Geometry: see drawing. Coordinates: mm, zero at the bounding-box minimum. Round coordinates to 2 decimals unless told otherwise and drop trailing zeros. Order: outer loops, then holes, each group sorted by start corner. A loop starts at its lowest first (then second) coordinate and runs counter-clockwise, first axis right, second up. Notation, with made-up numbers: (-15, 46) -> (22, 46) arc R37 ccw to (22, 85) -> close; hole circle Ø5 at (43.25, 38.25). An arc over 180 degrees is marked (long way). Put each result on its own line as item: value.
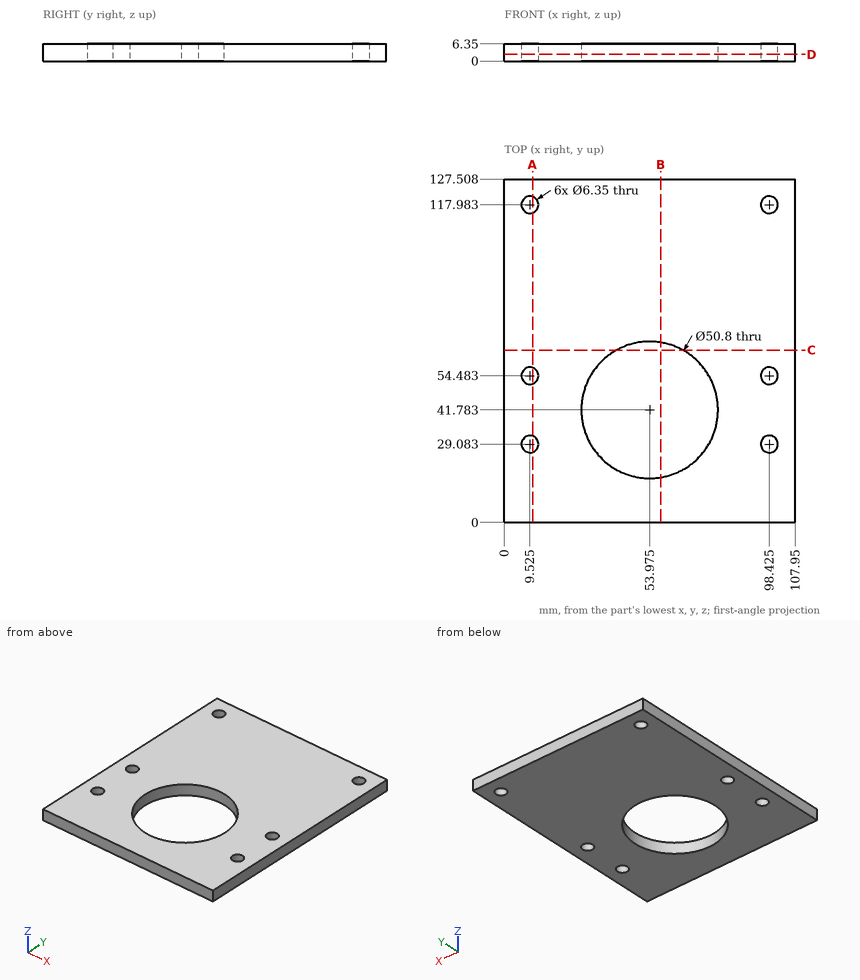
1. Cut plane B-B on x = 58. Return loops of the section in (y, z).
Ans:
outline: (0, 0) -> (16.7, 0) -> (16.7, 6.35) -> (0, 6.35) -> close; (66.86, 0) -> (127.51, 0) -> (127.51, 6.35) -> (66.86, 6.35) -> close
2. Cut plane C-C on y = 64. Return loops of the section in (x, z), and give its area (3 significant figures).
Ans:
outline: (0, 0) -> (41.66, 0) -> (41.66, 6.35) -> (0, 6.35) -> close; (66.29, 0) -> (107.95, 0) -> (107.95, 6.35) -> (66.29, 6.35) -> close
area: 529 mm²
3. Cut plane A-A on x = 10.5. Return loops of the section in (y, z), and give its area (3 significant figures).
Ans:
outline: (0, 0) -> (26.06, 0) -> (26.06, 6.35) -> (0, 6.35) -> close; (32.1, 0) -> (51.46, 0) -> (51.46, 6.35) -> (32.1, 6.35) -> close; (57.5, 0) -> (114.96, 0) -> (114.96, 6.35) -> (57.5, 6.35) -> close; (121, 0) -> (127.51, 0) -> (127.51, 6.35) -> (121, 6.35) -> close
area: 695 mm²
4. Material intervals for probe 1 along Y at (x, z) = (53.5, 4.5); probe 2 along Y at (x, z) = (100.5, 5); probe 3 along Y at (x, z) = (101, 5.75), sorted ascending.
Ans:
probe 1: 0 to 16.39, 67.18 to 127.51
probe 2: 0 to 26.68, 31.49 to 52.08, 56.89 to 115.58, 120.39 to 127.51
probe 3: 0 to 27.23, 30.94 to 52.63, 56.34 to 116.13, 119.84 to 127.51
5. Cut plane D-D on z = 2.5. Return loops of the section in (x, y) (3 decimals).
Ans:
outline: (0, 0) -> (107.95, 0) -> (107.95, 127.508) -> (0, 127.508) -> close; hole circle Ø6.35 at (9.525, 29.083); hole circle Ø6.35 at (9.525, 54.483); hole circle Ø6.35 at (9.525, 117.983); hole circle Ø50.8 at (53.975, 41.783); hole circle Ø6.35 at (98.425, 29.083); hole circle Ø6.35 at (98.425, 54.483); hole circle Ø6.35 at (98.425, 117.983)
